from build123d import *

# Parameters (mm, degrees)
SKIZZE1_R                       = 21.25
AUFSATZ_LINEAR_AUSTRAGEN1_DEPTH = 66.5
SKIZZE2_R                       = 8.75
AUFSATZ_LINEAR_AUSTRAGEN2_DEPTH = 4.5
SKIZZE3_R                       = 2.5
AUFSATZ_LINEAR_AUSTRAGEN3_DEPTH = 15
SKIZZE4_R                       = 2.15
SCHNITT_LINEAR_AUSTRAGEN1_DEPTH = 10
SKIZZE5_R                       = 15
AUFSATZ_LINEAR_AUSTRAGEN4_DEPTH = 5
AUFSATZ_LINEAR_START            = 13
SKIZZE6_R                       = 21.25
AUFSATZ_LINEAR_AUSTRAGEN5_DEPTH = 13


with BuildPart() as part:
    # Skizze1 → Aufsatz-Linear austragen1 (new body)
    with BuildSketch(Plane.XY):
        Circle(SKIZZE1_R)
    extrude(amount=AUFSATZ_LINEAR_AUSTRAGEN1_DEPTH)

    # Skizze2 → Aufsatz-Linear austragen2 (add)
    with BuildSketch(Plane.XY.offset(66.5)):
        Circle(SKIZZE2_R)
    extrude(amount=AUFSATZ_LINEAR_AUSTRAGEN2_DEPTH)

    # Skizze3 → Aufsatz-Linear austragen3 (add)
    with BuildSketch(Plane.XY.offset(71)):
        Circle(SKIZZE3_R)
    extrude(amount=AUFSATZ_LINEAR_AUSTRAGEN3_DEPTH)

    # Skizze4 → Schnitt-Linear austragen1 (cut)
    with BuildSketch(Plane.XY.offset(66.5)):
        with Locations((-14.5, 0)):
            Circle(SKIZZE4_R)
        with Locations((14.5, 0)):
            Circle(SKIZZE4_R)
    extrude(amount=-SCHNITT_LINEAR_AUSTRAGEN1_DEPTH, mode=Mode.SUBTRACT)

    # Skizze5 → Aufsatz-Linear austragen4 (add)
    with BuildSketch(Plane(origin=(0, 0, 0), x_dir=(-1, 0, 0), z_dir=(0, 0, -1))):
        Circle(SKIZZE5_R)
    extrude(amount=AUFSATZ_LINEAR_AUSTRAGEN4_DEPTH)

    # Skizze6 → Aufsatz-Linear austragen5 (add)
    with BuildSketch(Plane(origin=(0, 0, -5), x_dir=(-1, 0, 0), z_dir=(0, 0, -1)).offset(AUFSATZ_LINEAR_START)):
        with Locations(Location((0, 0, 0), (0, 0, 180))):
            Circle(SKIZZE6_R)
    extrude(amount=-AUFSATZ_LINEAR_AUSTRAGEN5_DEPTH)


solid = part.part
For this review, take the finished solid that the model builds, in its own axes (mm). A direction names the side the tool comes from. Round coordinates to 2 decimals unless told otherwise and drop trailing zeros. Loops run counter-clockwise (first coordinate to the right, second up) from the corner with the lowest first, then second, coordinate; pieces in that order, holes last. Notation, with made-up numbers: (55, -39) - (70, -39) arc R11 cw to (70, -19) - close; hole circle Ø7 at (84, -21). An arc over 180 degrees is marked (long way). Use one line per item in the form item = value.
1) We need section A-A on y = 17. Write out the cut boundary in (x, z), then the cut area to 3 significant figures.
Solutions:
outline = (-12.75, -18) - (12.75, -18) - (12.75, -5) - (-12.75, -5) - close; (-12.75, 0) - (12.75, 0) - (12.75, 66.5) - (-12.75, 66.5) - close
area = 2,030 mm2
2) We need section C-C on y = 0. Write out the cut boundary in (x, z), then the cut area to 3 significant figures.
Solutions:
outline = (-21.25, -18) - (21.25, -18) - (21.25, -5) - (15, -5) - (15, 0) - (21.25, 0) - (21.25, 66.5) - (16.65, 66.5) - (16.65, 56.5) - (12.35, 56.5) - (12.35, 66.5) - (8.75, 66.5) - (8.75, 71) - (2.5, 71) - (2.5, 86) - (-2.5, 86) - (-2.5, 71) - (-8.75, 71) - (-8.75, 66.5) - (-12.35, 66.5) - (-12.35, 56.5) - (-16.65, 56.5) - (-16.65, 66.5) - (-21.25, 66.5) - (-21.25, 0) - (-15, 0) - (-15, -5) - (-21.25, -5) - close
area = 3,600 mm2
3) We need section B-B on x = 0. Write out the cut boundary in (y, z), then the cut area to 3 significant figures.
Solutions:
outline = (-21.25, -18) - (21.25, -18) - (21.25, -5) - (15, -5) - (15, 0) - (21.25, 0) - (21.25, 66.5) - (8.75, 66.5) - (8.75, 71) - (2.5, 71) - (2.5, 86) - (-2.5, 86) - (-2.5, 71) - (-8.75, 71) - (-8.75, 66.5) - (-21.25, 66.5) - (-21.25, 0) - (-15, 0) - (-15, -5) - (-21.25, -5) - close
area = 3,680 mm2
4) Wall thickness on probe 1 along Z at (x, y) = (-4, 17); probe 2 along Z at (x, y) = (9, 11); probe 3 along Z at (x, y) = (0, -7.5): over which ranges is each line inside the solid? List them lowest first.
Solutions:
probe_1 = -18 to -5, 0 to 66.5
probe_2 = -18 to 66.5
probe_3 = -18 to 71
5) Mouldability with a two-part tool opening along X and no side actions: class faces 1 (the face through (4.4, -14.5, -5)), 2 (the face through (-6.944, -5.324, 68.718)), 3 (the face through (-15, 0, 56.5)) as pulls with the +X half, pulls with the -X half, needs draft (parallel to the pull), parting line crosses it, or undercut.
Solutions:
face_1 = needs draft
face_2 = parting line crosses it
face_3 = undercut
6) Clearance check with flat-ended pins moving along their axes: P1, Ø7, axis at x = -14.5, y = 0, coming from the +Z side; P2, Ø12, axis at x = 6, y = -11, coming from the +Z side; P3, Ø2, axis at x = -14.5, y = -0.5, coming from the +Z side. State where each tip first meets the part, or that it passes through.
Solutions:
P1 = 66.5
P2 = 71
P3 = 56.5
7) We need section D-D on z = -7.5. Write out the cut boundary in (x, y), then the cut area to 3 significant figures.
Solutions:
outline = circle Ø42.5 at (0, 0)
area = 1,420 mm2
8) Tool access review of faces 4 (the face through (16.55, 0.65, 61.57)), 5 (the face through (-14.5, -4.4, 0)), 6 (the face through (-16.863, -12.93, 32.784)): name each direction out of +Z, -Z, +X, -X, +Y, -Y from which nothing blocks a thin tool from reaching the whole face with its end or side.
Solutions:
face_4 = +Z
face_5 = none
face_6 = +Z, -Z
